```python
from build123d import *

# Parameters (mm, degrees)
SKETCH1_W                       = 131
SKETCH1_H                       = 98
SKETCH1_W_2                     = 125
SKETCH1_H_2                     = 90
BOSS_EXTRUDE1_DEPTH             = 80
SKETCH2_W                       = 131
SKETCH2_H                       = 98
BOSS_EXTRUDE2_DEPTH             = 3
SKETCH4_W                       = 125
SKETCH4_H                       = 90
SKETCH4_W_2                     = 119.5
SKETCH4_H_2                     = 84.5
BOSS_EXTRUDE3_DEPTH             = 3
SKETCH5_W                       = 15
SKETCH5_H                       = 73
CABLE_CUT_TOP_DEPTH             = 4
CABLE_CUT_BOTTOM_RIGHT_REACH    = 141.736
SKETCH6_W                       = 20
SKETCH6_H                       = 52
SKETCH10_W                      = 15
SKETCH10_H                      = 38
CABLE_CUT_BOTTOM_LEFT_DEPTH     = 4
SCHANIER_CUT_REACH              = 141.736
SKETCH7_W                       = 35
SKETCH7_H                       = 20
SKETCH8_W                       = 4
SKETCH8_H                       = 10
SCHANIER_DEPTH                  = 10
F_3D_PRINTER_SUPPORT_DEPTH      = 43
SKIZZE3_W                       = 35
SKIZZE3_H                       = 10
SCHNITT_LINEAR_AUSTRAGEN1_DEPTH = 20
SCHNITT_LINEAR_AUSTRAGEN3_REACH = 120.258
SKIZZE5_R                       = 1.75
AUFSATZ_LINEAR_AUSTRAGEN2_DEPTH = 25
SCHNITT_LINEAR_AUSTRAGEN4_REACH = 118.534
SKIZZE10_R                      = 2.1
CUT_EXTRUDE4_REACH              = 163.127


with BuildPart() as part:
    # Sketch1 → Boss-Extrude1 (new body)
    with BuildSketch(Plane(origin=(0, 0, 0), x_dir=(1, 0, 0), z_dir=(0, 1, 0))):
        Rectangle(SKETCH1_W, SKETCH1_H)
        Rectangle(SKETCH1_W_2, SKETCH1_H_2, mode=Mode.SUBTRACT)
    extrude(amount=BOSS_EXTRUDE1_DEPTH)

    # Sketch2 → Boss-Extrude2 (add)
    with BuildSketch(Plane.XZ):
        Rectangle(SKETCH2_W, SKETCH2_H)
    extrude(amount=BOSS_EXTRUDE2_DEPTH)

    # Sketch4 → Boss-Extrude3 (add)
    with BuildSketch(Plane(origin=(0, 0, 0), x_dir=(1, 0, 0), z_dir=(0, 1, 0))):
        Rectangle(SKETCH4_W, SKETCH4_H)
        with Locations((-0.25, 0.25)):
            Rectangle(SKETCH4_W_2, SKETCH4_H_2, mode=Mode.SUBTRACT)
    extrude(amount=BOSS_EXTRUDE3_DEPTH)

    # Sketch5 → Cable Cut Top (cut)
    with BuildSketch(Plane(origin=(0, 0, -49), x_dir=(-1, 0, 0), z_dir=(0, 0, -1))):
        with Locations((22.5, 43.5)):
            Rectangle(SKETCH5_W, SKETCH5_H)
    extrude(amount=-CABLE_CUT_TOP_DEPTH, mode=Mode.SUBTRACT)

    # Sketch6 → Cable Cut Bottom Right (cut, up to next)
    with BuildSketch(Plane(origin=(0, 0, 45), x_dir=(-1, 0, 0), z_dir=(0, 0, -1)), mode=Mode.PRIVATE) as cable_cut_bottom_right_sk1:
        with Locations((-37.5, 54)):
            Rectangle(SKETCH6_W, SKETCH6_H)
    cable_cut_bottom_right_tool1 = extrude(cable_cut_bottom_right_sk1.sketch, amount=-CABLE_CUT_BOTTOM_RIGHT_REACH, mode=Mode.PRIVATE) & part.part
    add(cable_cut_bottom_right_tool1.solids().sort_by_distance((37.5, 54, 45))[0], mode=Mode.SUBTRACT)

    # Sketch10 → Cable Cut Bottom Left (cut)
    with BuildSketch(Plane.XY.offset(49)):
        with Locations((-22.5, 61)):
            Rectangle(SKETCH10_W, SKETCH10_H)
    extrude(amount=-CABLE_CUT_BOTTOM_LEFT_DEPTH, mode=Mode.SUBTRACT)

    # Sketch7 → Schanier Cut (cut, up to next)
    with BuildSketch(Plane.XY.offset(-45), mode=Mode.PRIVATE) as schanier_cut_sk1:
        with Locations((28, 70)):
            Rectangle(SKETCH7_W, SKETCH7_H)
    schanier_cut_tool1 = extrude(schanier_cut_sk1.sketch, amount=-SCHANIER_CUT_REACH, mode=Mode.PRIVATE) & part.part
    add(schanier_cut_tool1.solids().sort_by_distance((28, 70, -45))[0], mode=Mode.SUBTRACT)

    # Sketch8 → Schanier (add)
    with BuildSketch(Plane.XY.offset(-45)):
        with Locations((8.5, 75)):
            Rectangle(SKETCH8_W, SKETCH8_H)
        with Locations((47.5, 75)):
            Rectangle(SKETCH8_W, SKETCH8_H)
    extrude(amount=SCHANIER_DEPTH)

    # Skizze2 → 3D Printer Support (add)
    with BuildSketch(Plane.ZY.offset(-6.5)):
        Polygon((-35, 70), (-45, 70), (-45, 58.082464074), align=None)
    extrude(amount=-F_3D_PRINTER_SUPPORT_DEPTH)

    # Skizze3 → Schnitt-Linear austragen1 (cut)
    with BuildSketch(Plane(origin=(0, 0, -45), x_dir=(-1, 0, 0), z_dir=(0, 0, -1))):
        with Locations((-28, 65)):
            Rectangle(SKIZZE3_W, SKIZZE3_H)
    extrude(amount=-SCHNITT_LINEAR_AUSTRAGEN1_DEPTH, mode=Mode.SUBTRACT)

    # Schnitt-Linear austragen3: up to this face of the body (flat: up to its plane)
    schnitt_linear_austragen3_end = Plane(part.part.faces().sort_by_distance((49.5, 71.649796712, -40.622308687))[0])
    # Skizze5 → Schnitt-Linear austragen3 (cut, up to the picked face)
    with BuildSketch(Plane.ZY.offset(-6.5), mode=Mode.PRIVATE) as schnitt_linear_austragen3_sk1:
        with Locations((-41, 76.645898034)):
            Circle(SKIZZE5_R)
    schnitt_linear_austragen3_tool1 = split(extrude(schnitt_linear_austragen3_sk1.sketch, amount=-SCHNITT_LINEAR_AUSTRAGEN3_REACH, mode=Mode.PRIVATE), bisect_by=schnitt_linear_austragen3_end, keep=Keep.BOTH, mode=Mode.PRIVATE)
    add(schnitt_linear_austragen3_tool1.solids().sort_by(Axis((6.5, 76.645898, -41), (1, 0, 0)))[0], mode=Mode.SUBTRACT)

    # Skizze9 → Aufsatz-Linear austragen2 (add)
    with BuildSketch(Plane(origin=(27.5, 0, 0), x_dir=(0, 0, -1), z_dir=(1, 0, 0))):
        Polygon((-45, 80), (-32, 80), (-32, 75), (-45, 64.091704795), align=None)
    extrude(amount=-AUFSATZ_LINEAR_AUSTRAGEN2_DEPTH)

    # Schnitt-Linear austragen4: up to this plane
    schnitt_linear_austragen4_end = Plane(origin=(2.5, 75, 32), z_dir=(0, -0.766044443118974, -0.6427876096865441))
    # Skizze10 → Schnitt-Linear austragen4 (cut, up to the surface)
    with BuildSketch(Plane(origin=(0, 80, 0), x_dir=(1, 0, 0), z_dir=(0, 1, 0)), mode=Mode.PRIVATE) as schnitt_linear_austragen4_sk1:
        with Locations(Location((20, -37, 0), (0, 0, 270))):
            Circle(SKIZZE10_R)
    schnitt_linear_austragen4_tool1 = split(extrude(schnitt_linear_austragen4_sk1.sketch, amount=-SCHNITT_LINEAR_AUSTRAGEN4_REACH, mode=Mode.PRIVATE), bisect_by=schnitt_linear_austragen4_end, keep=Keep.BOTH, mode=Mode.PRIVATE)
    add(schnitt_linear_austragen4_tool1.solids().sort_by_distance((20, 80, 37))[0], mode=Mode.SUBTRACT)

    # Cut-Extrude4: up to this face of the body (flat: up to its plane)
    cut_extrude4_end = Plane(part.part.faces().sort_by_distance((65.5, 38.5, 0))[0])
    # Sketch9 → Cut-Extrude4 (cut, up to the picked face)
    with BuildSketch(Plane.ZY.offset(65.5), mode=Mode.PRIVATE) as cut_extrude4_sk1:
        Polygon((-46, 78), (-46.5, 78), (-46.5, 75), (-47.25, 75), (-47.25, 68.5), (-49, 68.5), (-49, 80), (-46, 80), align=None)
    cut_extrude4_tool1 = split(extrude(cut_extrude4_sk1.sketch, amount=-CUT_EXTRUDE4_REACH, mode=Mode.PRIVATE), bisect_by=cut_extrude4_end, keep=Keep.BOTH, mode=Mode.PRIVATE)
    add(cut_extrude4_tool1.solids().sort_by(Axis((-65.5, 74.930905, -47.861181), (1, 0, 0)))[0], mode=Mode.SUBTRACT)


solid = part.part
```
Read the model definition and answer for the solid it produces. Units are mm, in the model's axes. A direction names the side the tool comes from. Give positions to 0.01 mm unless a question says otherwise; leave off trailing zeros. Write each loop counter-clockwise with the first axis right and the second up, starting at its lowest first coordinate (ties: lowest second). Pieces come first, ordered by that corner, then holes. Notation, with made-up numbers: M -16.75,39.25 L 17.25,39.25 A16 ccw 17.25,49.25 Z; hole C 9,-2.5 d8. An arc over 180 degrees is marked long. Put each result on its own line as item: value. Start each with the question number.
1. The part is cut by section D-D, the plane z = -41. Give the vertices of the cut face in (x, y).
2. The part is cut by section A-A, the plane z = 37. Give the vertices of the cut face in (x, y), and give its area (3 significant figures).
3. The part is cut by section C-C, the plane y = 18. Give the vertices of the cut face in (x, z).
4. Consider line 1 along Z through (x, y) = (5, 24); line 2 along X through (y, z) = (54, -7.5); line 3 along Y through (x, z) = (47, -41). Determine where each line is inside the solid, lowest interval first.
5. For a pull along Y with two mould halves and no side action, classify faces 1 (the flat face through (11, 80, 43)), 2 (the flat face through (-1, 1, 42)), 3 (the flat face through (15.18, 69.62, 38.41)), 4 (the flat face through (-62.5, 41, 1)) as released by +Y, released by -Y, zero draft, split by the parting line, or undercut.
6. Which of the six approach directions +Z, -Z, +X, -X, +Y, -Y give full straight-line access (tool end or side, diameter ignored) to faces 5 (the flat face through (2.5, 74, 40)), 6 (the flat face through (10.5, 70, -42)), 7 (the flat face through (-15, 61, 47))?
7. The part is cut by section B-B, the plane x = -8.5. Give the vertices of the cut face in (y, z).
8. Each of these flat-tipped pins is pushed along its axis until it touches: pin 1 Ø2 at (x, y) = (2, 70.5) entering from -Z; pin 2 Ø12 at (x, z) = (-50.5, 15.5) entering from +Y; pin 3 Ø1.6 at (x, y) = (52.5, 79.5) entering from -Z. Where does it stop, or does it pass through?
Final values:
1. outline: M -65.5,-3 L 65.5,-3 L 65.5,80 L 62.5,80 L 62.5,3 L 59.5,3 L 59.5,0 L -60,0 L -60,3 L -62.5,3 L -62.5,80 L -65.5,80 Z; M 6.5,62.85 L 10.5,62.85 L 10.5,74.9 L 6.5,74.9 Z; M 6.5,78.4 L 10.5,78.4 L 10.5,80 L 6.5,80 Z; M 45.5,62.85 L 49.5,62.85 L 49.5,74.9 L 45.5,74.9 Z; M 45.5,78.4 L 49.5,78.4 L 49.5,80 L 45.5,80 Z
2. outline: M -65.5,-3 L 65.5,-3 L 65.5,80 L 62.5,80 L 62.5,3 L 59.5,3 L 59.5,0 L -60,0 L -60,3 L -62.5,3 L -62.5,80 L -65.5,80 Z; M 2.5,70.8 L 17.9,70.8 L 17.9,80 L 2.5,80 Z; M 22.1,70.8 L 27.5,70.8 L 27.5,80 L 22.1,80 Z
2. area: 1,080 mm²
3. outline: M -65.5,-49 L -30,-49 L -30,-45 L -62.5,-45 L -62.5,45 L 62.5,45 L 62.5,-45 L -15,-45 L -15,-49 L 65.5,-49 L 65.5,49 L -65.5,49 Z
4. line 1: z = -49 to -45, 45 to 49
4. line 2: x = -65.5 to -62.5, 62.5 to 65.5
4. line 3: y = -3 to 0, 62.85 to 74.9, 78.4 to 80
5. face 1: released by +Y
5. face 2: undercut
5. face 3: undercut
5. face 4: zero draft
6. face 5: +Y
6. face 6: -Z, +Y
6. face 7: +Z, -Z, +Y
7. outline: M -3,-49 L 68.5,-49 L 68.5,-47.25 L 75,-47.25 L 75,-46.5 L 78,-46.5 L 78,-46 L 80,-46 L 80,-45 L 3,-45 L 3,-42.5 L 0,-42.5 L 0,42 L 3,42 L 3,45 L 80,45 L 80,49 L -3,49 Z
8. pin 1: stops at z = -47.25
8. pin 2: stops at y = 0
8. pin 3: stops at z = -46
